Check sheet for the modelled part. Datum: model origin and axes. Units: mm. Face numbers are marked on the shaded views. A direction names the side the tool comes from. Round coordinates to 2 decimals unless told otherwise and drop trailing zeros. Loops run counter-clockwise (first coordinate to the right, second up) from the corner with the lowest first, then second, coordinate; pieces in that order, holes last. Notation, with made-up numbers: (-9.75, 80.25) -> (34.25, 80.25) arc R19 ccw to (34.25, 84.25) -> close; hole circle Ø2 at (-25.75, -22). An arc over 180 degrees is marked (long way). Return JSON: item names as keys, results as strings.
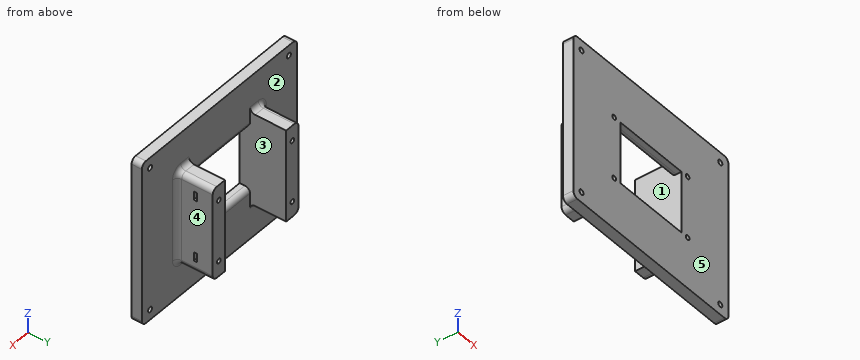
from build123d import *

# Parameters (mm, degrees)
SKETCH1_W           = 190
SKETCH1_H           = 160
BOSS_EXTRUDE1_DEPTH = 10
SKETCH3_W           = 15
SKETCH3_H           = 90
BOSS_EXTRUDE3_DEPTH = 35
SKETCH4_R           = 2.25
CUT_EXTRUDE1_DEPTH  = 50
SKETCH5_W           = 75
SKETCH5_H           = 60
CUT_EXTRUDE2_DEPTH  = 50
SKETCH8_R           = 2.5
CUT_EXTRUDE4_DEPTH  = 10
FILLET1_R           = 5
FILLET2_R           = 5
CUT_EXTRUDE5_DEPTH  = 3.3


with BuildPart() as part:
    # Sketch1 → Boss-Extrude1 (new body)
    with BuildSketch(Plane(origin=(0, 0, 0), x_dir=(1, 0, 0), z_dir=(0, 1, 0))):
        with Locations((95, 80)):
            Rectangle(SKETCH1_W, SKETCH1_H)
    extrude(amount=BOSS_EXTRUDE1_DEPTH)

    # Sketch3 → Boss-Extrude3 (add)
    with BuildSketch(Plane(origin=(0, 10, 0), x_dir=(1, 0, 0), z_dir=(0, 1, 0))):
        with Locations((50, 80)):
            Rectangle(SKETCH3_W, SKETCH3_H)
        with Locations((140, 80)):
            Rectangle(SKETCH3_W, SKETCH3_H)
    extrude(amount=BOSS_EXTRUDE3_DEPTH)

    # Sketch4 → Cut-Extrude1 (cut)
    with BuildSketch(Plane(origin=(0, 45, 0), x_dir=(1, 0, 0), z_dir=(0, 1, 0))):
        with Locations(Location((50, 110, 0), (0, 0, 270))):
            Circle(SKETCH4_R)
        with Locations(Location((140, 110, 0), (0, 0, 270))):
            Circle(SKETCH4_R)
        with Locations(Location((140, 50, 0), (0, 0, 270))):
            Circle(SKETCH4_R)
        with Locations(Location((50, 50, 0), (0, 0, 270))):
            Circle(SKETCH4_R)
    extrude(amount=-CUT_EXTRUDE1_DEPTH, mode=Mode.SUBTRACT)

    # Sketch5 → Cut-Extrude2 (cut)
    with BuildSketch(Plane(origin=(0, 10, 0), x_dir=(1, 0, 0), z_dir=(0, 1, 0))):
        with Locations((95, 80)):
            Rectangle(SKETCH5_W, SKETCH5_H)
    extrude(amount=-CUT_EXTRUDE2_DEPTH, mode=Mode.SUBTRACT)

    # Sketch8 → Cut-Extrude4 (cut)
    with BuildSketch(Plane(origin=(0, 10, 0), x_dir=(1, 0, 0), z_dir=(0, 1, 0))):
        with Locations(Location((10, 150, 0), (0, 0, 270))):
            Circle(SKETCH8_R)
        with Locations(Location((180, 150, 0), (0, 0, 270))):
            Circle(SKETCH8_R)
        with Locations(Location((180, 10, 0), (0, 0, 270))):
            Circle(SKETCH8_R)
        with Locations(Location((10, 10, 0), (0, 0, 270))):
            Circle(SKETCH8_R)
    extrude(amount=-CUT_EXTRUDE4_DEPTH, mode=Mode.SUBTRACT)

    # Fillet1
    fillet1_edges = [part.edges().sort_by_distance(p)[0] for p in [
        (50, 10, -125),
        (42.5, 10, -80),
        (42.5, 27.5, -125),
        (50, 10, -35),
        (42.5, 27.5, -35),
        (147.5, 10, -80),
        (147.5, 27.5, -35),
        (140, 10, -125),
        (147.5, 27.5, -125),
        (140, 10, -35),
        (0, 5, -160),
        (190, 5, -160),
        (190, 5, 0),
        (0, 5, 0),
    ]]
    fillet(fillet1_edges, radius=FILLET1_R)

    # Fillet2
    fillet2_edges = [part.edges().sort_by_distance(p)[0] for p in [
        (95, 10, -50),
        (95, 10, -110),
    ]]
    fillet(fillet2_edges, radius=FILLET2_R)

    # Sketch10 → Cut-Extrude5 (cut)
    with BuildSketch(Plane(origin=(0, 30, 0), x_dir=(1, 0, 0), z_dir=(0, 1, 0))):
        Polygon((45.851380251, 54.148619749), (42.5, 54.148619749), (42.5, 45.848619749), (45.845857409, 45.848619749), (54.151380251, 45.848619749), (54.151380251, 54.148619749), align=None)
        Polygon((42.5, 105.848619749), (45.845857409, 105.848619749), (54.151380251, 105.848619749), (54.151380251, 114.148619749), (45.851380251, 114.148619749), (42.5, 114.148619749), align=None)
        Polygon((147.5, 45.848619749), (144.154142591, 45.848619749), (135.848619749, 45.848619749), (135.848619749, 54.148619749), (144.148619749, 54.148619749), (147.5, 54.148619749), align=None)
        Polygon((147.5, 114.148619749), (147.5, 105.848619749), (144.154142591, 105.848619749), (135.848619749, 105.848619749), (135.848619749, 114.148619749), (144.148619749, 114.148619749), align=None)
    extrude(amount=-CUT_EXTRUDE5_DEPTH, mode=Mode.SUBTRACT)


solid = part.part
Q1. Material ranges on line 1 (X direction, y = 34.5, z = -50); line 2 (Z direction, x = 140, y = 36); line 3 (Z direction, x = 140, y = 8), recorded low to high.
Results list:
{"line 1": "42.5 to 47.75, 52.25 to 57.5, 132.5 to 137.75, 142.25 to 147.5", "line 2": "-125 to -112.25, -107.75 to -52.25, -47.75 to -35", "line 3": "-160 to -112.25, -107.75 to -52.25, -47.75 to 0"}
Q2. Section check C-C (x = 94.5). Record the boundary of the cut face in (y, z).
Results list:
{"outline": "(0, -160) -> (10, -160) -> (10, -115) arc R5 ccw to (5, -110) -> (0, -110) -> close; (0, -50) -> (5, -50) arc R5 ccw to (10, -45) -> (10, 0) -> (0, 0) -> close"}
Q3. Section check A-A (x = 50). Count the separate pieces of the cut face and the enclosed holes in it, then the cut area to 3 significant figures.
Results list:
{"separate pieces": "3", "enclosed holes": "0", "area": "4,330 mm^2"}
Q4. Tool access check on the marked faces 3, 4 and 5. Record the directions out of +Z, -Z, +X, -X, +Y, -Y that give a thin tool (end or side, any length) a straight path to the whole face; none if there is none.
Results list:
{"face 3": "+Y", "face 4": "+Z, -Z, +X, +Y", "face 5": "+Z, -Z, +X, -X, -Y"}
Q5. Section check B-B (y = 23). Record the boundary of the cut face in (x, z), then the cut area to 3 significant figures.
Results list:
{"outline": "(42.5, -120) arc R5 ccw to (47.5, -125) -> (57.5, -125) -> (57.5, -35) -> (47.5, -35) arc R5 ccw to (42.5, -40) -> close; (132.5, -125) -> (142.5, -125) arc R5 ccw to (147.5, -120) -> (147.5, -40) arc R5 ccw to (142.5, -35) -> (132.5, -35) -> close; hole circle Ø4.5 at (50, -110); hole circle Ø4.5 at (50, -50); hole circle Ø4.5 at (140, -110); hole circle Ø4.5 at (140, -50)", "area": "2,610 mm^2"}
Q6. Draft check along Z on the marked faces 1 and 2. Enter one of: released by +Z, released by -Z, zero draft, split by the parting line, or undercut.
Results list:
{"face 1": "undercut", "face 2": "zero draft"}
Q7. Section check D-D (x = 10). Record the boundary of the cut face in (y, z), then the cut area to 3 significant figures.
Results list:
{"outline": "(0, -160) -> (10, -160) -> (10, -152.5) -> (0, -152.5) -> close; (0, -147.5) -> (10, -147.5) -> (10, -12.5) -> (0, -12.5) -> close; (0, -7.5) -> (10, -7.5) -> (10, 0) -> (0, 0) -> close", "area": "1,500 mm^2"}
Q8. Go/stop test with flat-tipped pins: pin 1 (3.5 mm diameter, centred on y = 28, z = -109.5, fed in from +X); pin 2 (1 mm diameter, centred on x = 143.5, y = 28, fed in from -Z); pin 3 (3.5 mm diameter, centred on y = 29, z = -51, fed in from -X). Record where each tip stops, or that it passes through.
Results list:
{"pin 1": "x = 147.5", "pin 2": "z = -124.97", "pin 3": "x = 42.5"}
